For this review, take the finished solid that the model builds, in its own axes (mm). Face numbers are marked on the shaded views. A direction names the side the tool comes from. Coordinates: 2 decimals unless noted, no trailing zeros. Write each loop counter-clockwise with the first axis right and the second up, starting at its lowest first coordinate (ties: lowest second). Pieces come first, ordered by that corner, then holes. Notation, with made-up numbers: (8, -17) -> (36, -17) arc R30 ccw to (36, 12) -> close; hole circle Ø6 at (86, 81). An arc over 180 degrees is marked (long way). One line per item, written item: value. Start each with the question number.
1) For probe 1 along X at (y, z) = (2, -16.51); probe 2 along Z at (x, y) = (38.1, 5.25); probe 3 along X at (y, z) = (1.75, -14), list the stretches that pass through material, from the lowest coordinate up. Write a range as from..to.
2) For pin 1 Ø1.5 at (x, z) = (13, -14) entering from +Y; pin 2 Ø1.9 at (y, z) = (15, -31) entering from +X; pin 3 Ø4 at (y, z) = (16.5, -8.5) entering from +X, all flat-tipped, find the tip position at first contact; note any pin that passes through.
3) Add section C-C (y = 9.5). State the section outline as (x, z) points.
4) Mouldability with a two-part tool opening along Z and no side actions: class the marked faces 1, 2, 3 and 4 as released by +Z, released by -Z, zero draft, split by the parting line, or undercut.
5) Machinability: for the marked faces 5, 6 and 7, which of the approach directions +Z, -Z, +X, -X, +Y, -Y give a long, thin tool a straight path to every point of the face, cutting with its end or side? Answer none if there is none.
6) Add section A-A (x = 38.1). State the section outline as (y, z) points.
7) Add section D-D (y = 5). State the section outline as (x, z) points.
8) Add section B-B (z = -16.51). State the section outline as (x, y) points, and give its area (3 significant figures).
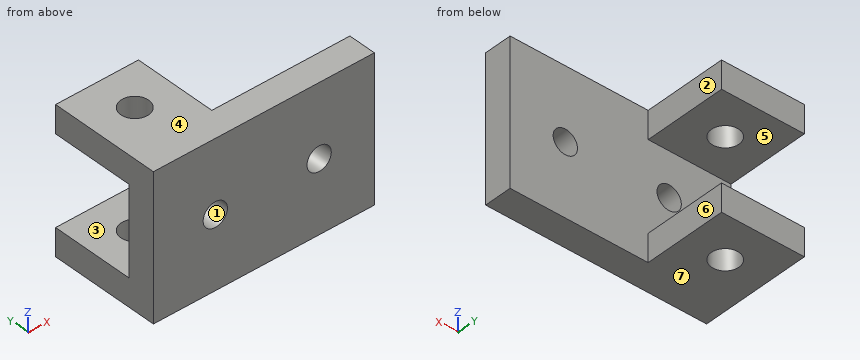
from build123d import *

# Parameters (mm, degrees)
SKETCH3_W           = 50.8
SKETCH3_H           = 33.02
BOSS_EXTRUDE2_DEPTH = 6.35
SKETCH4_R           = 2.794
CUT_EXTRUDE1_DEPTH  = 7.35
SKETCH5_W           = 19.05
SKETCH5_H           = 6.35
BOSS_EXTRUDE3_DEPTH = 19.05
SKETCH7_R           = 3.175
CUT_EXTRUDE2_DEPTH  = 34.29


with BuildPart() as part:
    # Sketch3 → Boss-Extrude2 (new body)
    with BuildSketch(Plane(origin=(0, 0, 0), x_dir=(1, 0, 0), z_dir=(0, 1, 0))):
        with Locations((25.4, 16.51)):
            Rectangle(SKETCH3_W, SKETCH3_H)
    extrude(amount=BOSS_EXTRUDE2_DEPTH)

    # Sketch4 → Cut-Extrude1 (cut, through all)
    with BuildSketch(Plane(origin=(0, 6.35, 0), x_dir=(1, 0, 0), z_dir=(0, 1, 0))):
        with Locations((14.224, 16.51)):
            Circle(SKETCH4_R)
        with Locations((38.1, 16.51)):
            Circle(SKETCH4_R)
    extrude(amount=-CUT_EXTRUDE1_DEPTH, mode=Mode.SUBTRACT)

    # Sketch5 → Boss-Extrude3 (add)
    with BuildSketch(Plane(origin=(0, 6.35, 0), x_dir=(1, 0, 0), z_dir=(0, 1, 0))):
        with Locations((9.525, 3.175)):
            Rectangle(SKETCH5_W, SKETCH5_H)
    boss_extrude3 = extrude(amount=BOSS_EXTRUDE3_DEPTH)

    # Mirror1: Boss-Extrude3 across plane
    add(boss_extrude3.mirror(Plane.XY.offset(-16.51)))

    # Sketch7 → Cut-Extrude2 (cut)
    with BuildSketch(Plane.XY):
        with Locations((9.652, 15.748)):
            Circle(SKETCH7_R)
    extrude(amount=-CUT_EXTRUDE2_DEPTH, mode=Mode.SUBTRACT)


solid = part.part
Numbers:
1. probe 1: 0..11.43, 17.02..35.31, 40.89..50.8
1. probe 2: -33.02..-19.3, -13.72..0
1. probe 3: 0..13, 15.45..36.87, 39.33..50.8
2. pin 1: y = 6.35
2. pin 2: x = 19.05
2. pin 3: through
3. outline: (0, -33.02) -> (19.05, -33.02) -> (19.05, -26.67) -> (0, -26.67) -> close; (0, -6.35) -> (19.05, -6.35) -> (19.05, 0) -> (0, 0) -> close
4. face 1: undercut
4. face 2: zero draft
4. face 3: undercut
4. face 4: released by +Z
5. face 5: +X, -X, +Y
5. face 6: +Z, -Z, +X, +Y
5. face 7: -Z, +X, -X, +Y, -Y
6. outline: (0, -33.02) -> (6.35, -33.02) -> (6.35, -19.3) -> (0, -19.3) -> close; (0, -13.72) -> (6.35, -13.72) -> (6.35, 0) -> (0, 0) -> close
7. outline: (0, -33.02) -> (50.8, -33.02) -> (50.8, 0) -> (0, 0) -> close; hole circle Ø5.59 at (14.22, -16.51); hole circle Ø5.59 at (38.1, -16.51)
8. outline: (0, 0) -> (11.43, 0) -> (11.43, 6.35) -> (0, 6.35) -> close; (17.02, 0) -> (35.31, 0) -> (35.31, 6.35) -> (17.02, 6.35) -> close; (40.89, 0) -> (50.8, 0) -> (50.8, 6.35) -> (40.89, 6.35) -> close
8. area: 252 mm²
